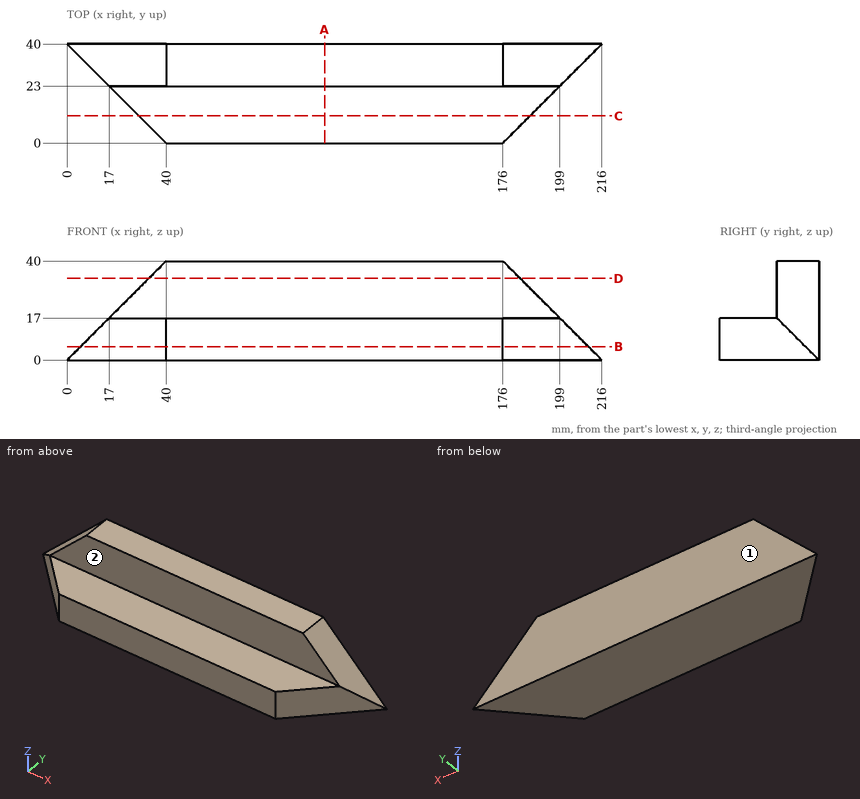
Design review of the part shown in the three views and the two pictorial views. Dimensions are in mm from the part's minimum x, y and z. A direction names the side the tool comes from. Round coordinates to 2 decimals unless told otherwise and drop trailing zeros. Write each loop counter-clockwise with the first axis right and the second up, starting at its lowest first coordinate (ties: lowest second). Pieces come first, ordered by that corner, then holes. Notation, with made-up numbers: (-21.5, -35) - (5.5, -35) arc R23 ccw to (5.5, -11) - close; hole circle Ø8 at (-33, -4.5). An arc over 180 degrees is marked (long way). Answer as CSV lines item,"result". Start each with the question number.
(1) For pin 1 (7 mm diameter, centred on x = 101, y = 12.5, fed in from +Z); pin 2 (12 mm diameter, centred on y = 21.5, z = 11, fed in from +X); pin 3 (6 mm diameter, centred on x = 35.5, y = 21, fed in from +Z), all flat-tipped, find the tip position at first contact; note any pin that passes through.
(2) Machinability: for the marked faces 1 and 2, which of the approach directions +Z, -Z, +X, -X, +Y, -Y give a long, thin tool a straight path to every point of the face, cutting with its end or side? Answer none if there is none.
(3) Add section A-A, the plane x = 104. State the section outline as (y, z) points.
(4) For line 1 (Y direction, x = 124, z = 33); line 2 (Z direction, x = 73, y = 2); line 3 (X direction, y = 24, z = 10.5), list the stretches that pass through material, from the lowest coordinate up.
(5) Add section D-D, the plane z = 33. State the section outline as (x, y) points, plus the area to 3 significant figures.
(6) Add section B-B, the plane z = 5.5. State the section outline as (x, y) points.
(7) Add section C-C, the plane y = 11. State the section outline as (x, z) points.
From the geometry:
1,pin 1,"stops at z = 17"
1,pin 2,"stops at x = 203.5"
1,pin 3,"stops at z = 37.74"
2,face 1,"+Z, -Z, +X, -X, +Y"
2,face 2,"+Z, +X, -X, -Y"
3,outline,"(0, 0) - (40, 0) - (40, 40) - (23, 40) - (23, 17) - (0, 17) - close"
4,line 1,"y = 23 to 40"
4,line 2,"z = 0 to 17"
4,line 3,"x = 16 to 200"
5,outline,"(33, 23) - (183, 23) - (183, 40) - (33, 40) - close"
5,area,"2,550 mm²"
6,outline,"(5.5, 34.5) - (40, 0) - (176, 0) - (210.5, 34.5) - (210.5, 40) - (5.5, 40) - close"
7,outline,"(29, 0) - (187, 0) - (187, 17) - (29, 17) - close"
